Source: CAD feature listing. Evaluate the final solid. Frame: model axes, mm. Face numbers are marked on the shaded views. Coordinates: 2 decimals unless noted, no trailing zeros. Write each loop counter-clockwise with the first axis right and the second up, starting at its lowest first coordinate (ties: lowest second). Pieces come first, ordered by that corner, then holes. Notation, with made-up numbers: M 88.5,74 L 136.5,74 A21 ccw 136.5,113 Z; hole C 51,36.5 d6. An arc over 180 degrees is marked long. One line per item, written item: value. Start each with the question number.
Item 1: Cut plane D-D, the plane x = -0.5. Output: boundary loops of the cut face in (y, z), then the cut area to 3 significant figures.
Item 2: Mould query, pull axis X, two halves, no side actions, for the marked faces 1, 2, 3 and 4. Classes: released by +X, released by -X, zero draft, split by the parting line, or undercut.
Item 3: Pin query (flat end, axial travel): P1, Ø8, axis at x = 2.5, z = -2, coming from the +Y side; P2, Ø10, axis at y = 12, z = 12.5, coming from the +X side; P3, Ø6, axis at x = 0, y = 5, coming from the +Z side; P4, Ø10, axis at x = 10, z = -9.5, coming from the +Y side. Return the tip coordinate at first contact, or that it passes through.
Item 4: Ray query, L1, parallel to Y at x = -7.5, z = 12.5; L2, parallel to X at y = 9.75, z = 8; L3, parallel to X at y = 4.25, z = -15.5. Return the intervals inside material, ascending. Write a range as from..to.
Item 5: Cut plane C-C, the plane z = -2. Output: boundary loops of the cut face in (x, y).
Item 6: Cut plane B-B, the plane y = 2.5. Output: boundary loops of the cut face in (x, z), then the cut area to 3 significant figures.
Item 7: Cut plane A-A, the plane z = 11. Output: boundary loops of the cut face in (x, y), then the cut area to 3 significant figures.
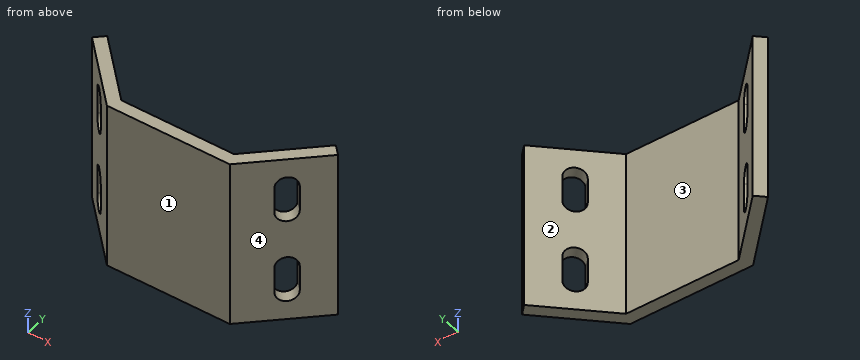
```python
from build123d import *

# Parameters (mm, degrees)
EXTRUDE_1_DEPTH     = 20
CUT_EXTRUDE_1_DEPTH = 14.621320344


with BuildPart() as part:
    # Эскиз1 → Вытянуть-Тонкостенный1 (new body)
    with BuildSketch(Plane.XY):
        Polygon((-27.878679656, 14.142135624), (-13.736544033, 0), (13.736544033, 0), (27.878679656, 14.142135624), (30, 12.02081528), (14.97918472, -3), (-14.97918472, -3), (-30, 12.02081528), align=None)
    extrude(amount=EXTRUDE_1_DEPTH)

    # Эскиз2 → Вырез-Вытянуть1 (cut, through all)
    with BuildSketch(Plane(origin=(-6.868272016, -6.868272016, 0), x_dir=(0, 0, -1), z_dir=(0.707106781, 0.707106781, 0))):
        with BuildLine():
            Line((-7, 17.213203436), (-13, 17.213203436))
            ThreePointArc((-13, 17.213203436), (-15.5, 19.713203436), (-13, 22.213203436))
            Line((-13, 22.213203436), (-7, 22.213203436))
            ThreePointArc((-7, 22.213203436), (-4.5, 19.713203436), (-7, 17.213203436))
        make_face()
    cut_extrude_1 = extrude(amount=-CUT_EXTRUDE_1_DEPTH, mode=Mode.SUBTRACT)

    # Зеркальное отражение1: Вырез-Вытянуть1 across plane
    add(cut_extrude_1.mirror(Plane(origin=(0, 0, 0), x_dir=(0, 0, 1), z_dir=(1, 0, 0))), mode=Mode.SUBTRACT)

    # Зеркальное отражение2: part across plane


with BuildPart() as part_1:
    add(part.part)
    add(part.part.mirror(Plane(origin=(0, 0, 0), x_dir=(1, 0, 0), z_dir=(0, 0, -1))))


solid = part_1.part
```
From the geometry:
1. outline: M -3,-20 L 0,-20 L 0,20 L -3,20 Z
1. area: 120 mm²
2. face 1: zero draft
2. face 2: undercut
2. face 3: undercut
2. face 4: released by +X
3. P1: stops at y = 0
3. P2: stops at x = 30
3. P3: passes through
3. P4: stops at y = 1.26
4. L1: y = -3..0
4. L2: x = -27.73..-23.49, 23.49..27.73
4. L3: x = -22.23..-17.99, 17.99..22.23
5. outline: M -30,12.02 L -14.98,-3 L 14.98,-3 L 30,12.02 L 27.88,14.14 L 13.74,0 L -13.74,0 L -27.88,14.14 Z
6. outline: M -20.48,-20 L -16.24,-20 L -16.24,20 L -20.48,20 Z; M 16.24,-20 L 20.48,-20 L 20.48,20 L 16.24,20 Z
6. area: 339 mm²
7. outline: M -30,12.02 L -24.7,6.72 L -22.58,8.84 L -27.88,14.14 Z; M -21.16,3.18 L -14.98,-3 L 14.98,-3 L 21.16,3.18 L 19.04,5.3 L 13.74,0 L -13.74,0 L -19.04,5.3 Z; M 22.58,8.84 L 24.7,6.72 L 30,12.02 L 27.88,14.14 Z
7. area: 180 mm²
